Model file for the job. Use its own axes, mm. A direction names the side the tool comes from. Give positions to 0.01 mm unless a question says otherwise; leave off trailing zeros. Order: outer loops, then holes, each group sorted by start corner. A loop starts at its lowest first (then second) coordinate and runs counter-clockwise, first axis right, second up. Notation, with made-up numbers: (-16, 29.25) - (10, 29.25) arc R24 cw to (10, 63.25) - close; hole circle Ø11 at (35.5, 89). An arc over 180 degrees is marked (long way). Use CSV: the item, a comma, the result in double quotes. Start each with the question number.
(1) Probe L1, parallel to X at y = -70.5, z = -8.5; L2, parallel to Y at x = 80.5, z = -5.25; L3, parallel to X at y = -58.5, z = -10.25. List the from-to ranges inside material, lowest first.
(2) Tool access for faces 1 (the flat face through (60, 61, 0)), 2 (the flat face through (19.05, -101, -6)): list every direction of +Z, -Z, +X, -X, +Y, -Y with a clear straight run to the whole face (end or side of a thin tool).
(3) Drop flat-ended pins along their axis: pin 1 Ø4 at (y, z) = (-89, -7) entering from +X; pin 2 Ø4 at (y, z) = (57.5, -9) entering from +X; pin 3 Ø2 at (x, z) = (24.5, -11) entering from -Y. Give the stop position or say it passes through.
(4) Band-saw the part on C-C, the plane x = 118.5. Give the cut face in (y, z).
(5) Band-saw the part on B-B, the plane y = -109.5. Give the cut face in (x, z).
(6) Band-saw the part on A-A, the plane z = -10. Give the cut face in (x, y).
Autodesk Inventor part; units mm, degrees
ref_plane "YZ Plane" through (0, 0, 0) normal (1, 0, 0) x (0, 1, 0)
ref_plane "XZ Plane" through (0, 0, 0) normal (0, 1, 0) x (-1, 0, 0)
ref_plane "XY Plane" through (0, 0, 0) normal (0, 0, 1) x (1, 0, 0)
sketch "Sketch1" plane through (0, 0, 0) normal (0, 0, 1) x (1, 0, 0)
  line L0 (6.35, -132.5) -> (19.05, -132.5)
  line L1 (19.05, 132.5) -> (6.35, 132.5)
  line L2 (6.35, 132.5) -> (6.35, -132.5)
  line L3 (146.05, 111.3788) -> (146.05, 132.5)
  line L4 (146.05, 132.5) -> (19.05, 132.5)
  line L5 (146.05, 111.3788) -> (19.05, -68.2625)
  line L6 (19.05, -132.5) -> (19.05, -68.2625)
  point P0 (0, 0)
extrude "Extrusion1" add sketch "Sketch1" against normal blind 12.7
properties part number "Side"
Answer block:
1,L1,"x = 6.35 to 19.05"
1,L2,"y = 18.66 to 132.5"
1,L3,"x = 6.35 to 25.95"
2,face 1,"+Z, +X, -X, +Y, -Y"
2,face 2,"+Z, -Z, +X, -Y"
3,pin 1,"stops at x = 19.05"
3,pin 2,"stops at x = 109.37"
3,pin 3,"stops at y = -61.97"
4,outline,"(72.41, -12.7) - (132.5, -12.7) - (132.5, 0) - (72.41, 0) - close"
5,outline,"(6.35, -12.7) - (19.05, -12.7) - (19.05, 0) - (6.35, 0) - close"
6,outline,"(6.35, -132.5) - (19.05, -132.5) - (19.05, -68.26) - (146.05, 111.38) - (146.05, 132.5) - (6.35, 132.5) - close"
